Could you check a few things on this drawing? It's one solid part, dimensions in mm from its lowest x, y, z. A direction names the side the tool comes from. Give positions to 0.01 mm unless a question says otherwise; leave off trailing zeros. Order: outer loops, then holes, each group sorted by start corner. A loop starts at its lowest first (then second) coordinate and runs counter-clockwise, first axis right, second up. Notation, with made-up numbers: M -5,85.5 L 39,85.5 A24 cw 39,106.5 Z; hole C -29.75,77 d1. An arc over 180 degrees is marked long. Use one line per item in the form item = value.
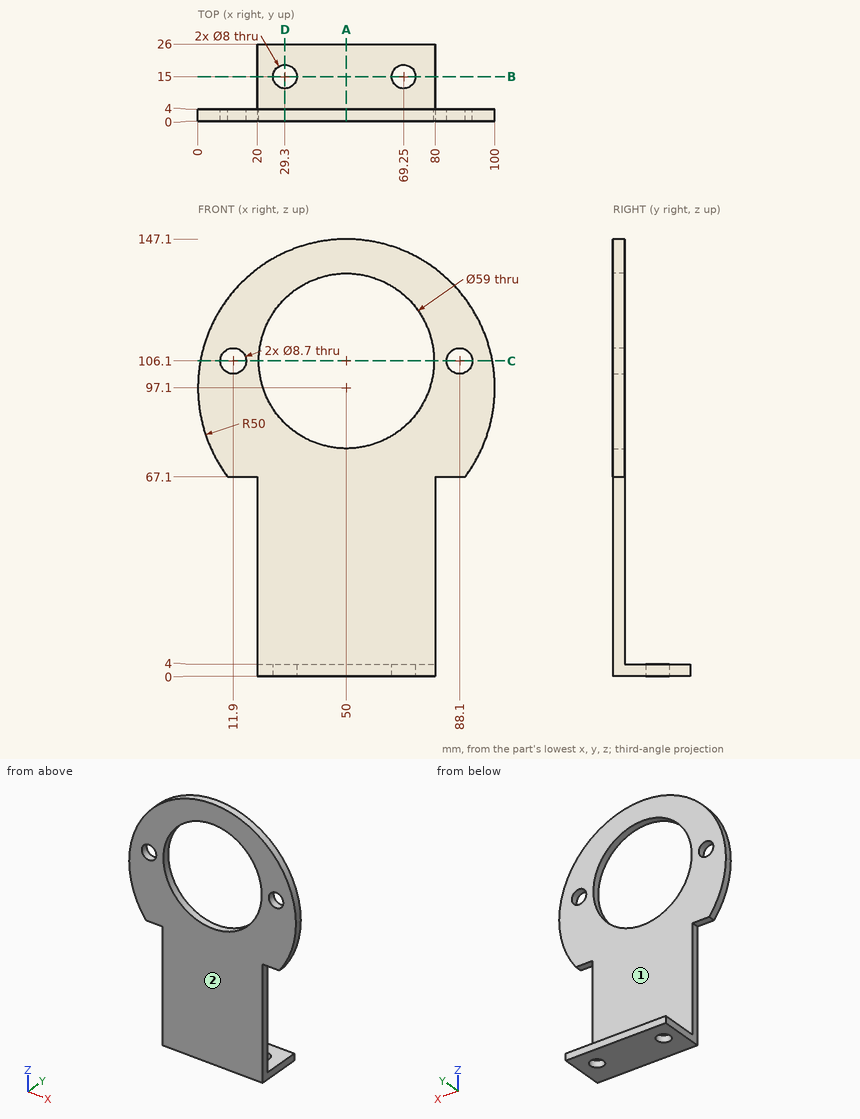
Q1. I'm going to push flat-ended pins straight in: pin 1 Ø6.5 at (x, y) = (29.3, 15) entering from -Z; pin 2 Ø6 at (x, y) = (72, 9.5) entering from +Z; pin 3 Ø2 at (x, y) = (15.5, 3) entering from -Z; pin 4 Ø8 at (y, z) = (7, 29.5) entering from +X. Where does each tip first touch, or does it pass through?
Found:
pin_1 = through
pin_2 = 4
pin_3 = 67.1
pin_4 = 80
Q2. I want a section at A-A on x = 50. Write out the boundary of the cut face in (y, z).
Found:
outline = M 0,0 L 26,0 L 26,4 L 4,4 L 4,76.6 L 0,76.6 Z; M 0,135.6 L 4,135.6 L 4,147.1 L 0,147.1 Z
Q3. I want a section at B-B on y = 15. Write out the boundary of the cut face in (x, z).
Found:
outline = M 20,0 L 25.3,0 L 25.3,4 L 20,4 Z; M 33.3,0 L 65.25,0 L 65.25,4 L 33.3,4 Z; M 73.25,0 L 80,0 L 80,4 L 73.25,4 Z
Q4. I want a section at D-D on x = 29.3. Write out the boundary of the cut face in (y, z), then the cut area to 3 significant figures.
Found:
outline = M 0,0 L 11,0 L 11,4 L 4,4 L 4,85.08 L 0,85.08 Z; M 0,127.12 L 4,127.12 L 4,142.61 L 0,142.61 Z; M 19,0 L 26,0 L 26,4 L 19,4 Z
area = 458 mm²
Q5. On a 3-axis mill with a long thin cutter (end or side, diameter ignored), from which of +Z, -Z, +X, -X, +Y, -Y can I reach the whole of each face in a straight line? I mean the marked faces 1 and 2. Say none if no direction works.
Found:
face_1 = +Z, +X, -X, +Y
face_2 = +Z, -Z, +X, -X, -Y
Q6. I need wall thicknesses on L1, parallel to X at y = 1.2, z = 106.1; L2, parallel to Y at x = 74.5, z = 75.5. Which ranges of each line are inside material? Lowest first, please.
Found:
L1 = 0.82 to 7.55, 16.25 to 20.5, 79.5 to 83.75, 92.45 to 99.18
L2 = 0 to 4
Q7. I want a section at C-C on z = 106.1. Write out the boundary of the cut face in (x, y), then the cut area to 3 significant figures.
Found:
outline = M 0.82,0 L 7.55,0 L 7.55,4 L 0.82,4 Z; M 16.25,0 L 20.5,0 L 20.5,4 L 16.25,4 Z; M 79.5,0 L 83.75,0 L 83.75,4 L 79.5,4 Z; M 92.45,0 L 99.18,0 L 99.18,4 L 92.45,4 Z
area = 87.9 mm²
